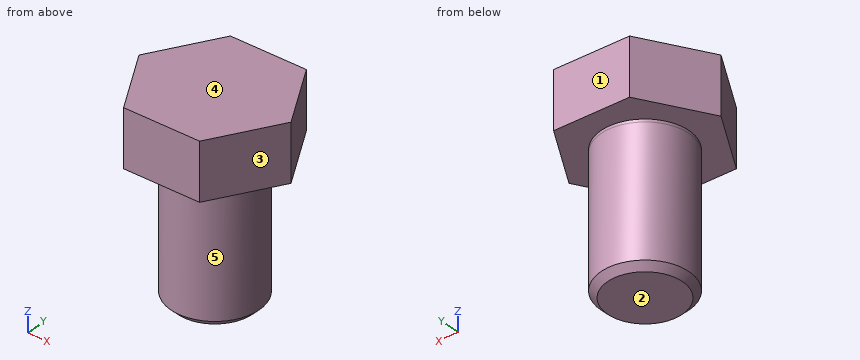
Solid Edge part; units mm, degrees
sketch "Sketch1" plane through (0, 0, 0) normal (0, 0, 1) x (1, 0, 0)
  circle A0 centre (0, 0) radius 13.92
extrude "Protrusion1" add sketch "Sketch1" along normal blind 10.32
sketch "Sketch2" plane through (0, 0, 0) normal (0, 0, -1) x (1, 0, 0)
  circle A0 centre (0, 0) radius 8
extrude "Protrusion2" add sketch "Sketch2" along normal blind 25
sketch "Sketch3" plane through (0, 0, -25) normal (0, 0, -1) x (1, 0, 0)
  circle A0 centre (0, 0) radius 7.9997
extrude "Cutout1" cut sketch "Sketch3" against normal blind 24.5 flip side to cut
chamfer "Chamfer_1" distance 1.2 angle 45 1 edges at (-7.9997, 0, -25)
sketch "Sketch4" plane through (0, 0, 10.32) normal (0, 0, 1) x (1, 0, 0)
  line L0 (-7.0545, 12) -> (7.0545, 12)
extrude "Cutout2" cut sketch "Sketch4" against normal up to next material side at (0, 12.05, 10.32)
pattern_circular "Pattern1" count 6 over 360 about axis through (0, 0, 10.32) along (0, 0, 1) of "Cutout2"
properties part number "118416" material "Stainless Steel, 304"
Input: part model. Units: mm. Frame: model coordinates. Face numbers are marked on the shaded views. A direction names the side the tool comes from. Coordinates: 2 decimals unless noted, no trailing zeros. Loops run counter-clockwise (first coordinate to the right, second up) from the corner with the lowest first, then second, coordinate; pieces in that order, holes last. Notation, with made-up numbers: (-28, 62.25) - (-3, 62.25) arc R14 cw to (-3, 84.25) - close; hole circle Ø4 at (31, 13). An arc over 180 degrees is marked (long way). Answer in a Markdown table with one row per item.
(1) Cut plane C-C on y = -9. Output: boundary loops of the cut face in (x, z), plus the area to 3 significant figures.
Model answer:
| item | result |
|---|---|
| outline | (-8.66, 0) - (8.66, 0) - (8.66, 10.32) - (-8.66, 10.32) - close |
| area | 179 mm² |
(2) Set-up query: the marked faces 4 and 5. Return all of +Z, -Z, +X, -X, +Y, -Y with unobstructed straight access to the full face (end or side cutting, diameter ignored); none if empty.
Model answer:
| item | result |
|---|---|
| face 4 | +Z, +X, -X, +Y, -Y |
| face 5 | -Z |
(3) Cut plane D-D on z = -4. Output: boundary loops of the cut face in (x, y), plus the area to 3 significant figures.
Model answer:
| item | result |
|---|---|
| outline | circle Ø16 at (0, 0) |
| area | 201 mm² |
(4) Pin query (flat end, axial travel): P1, Ø3, axis at y = -5, z = 2.5, coming from the +X side; P2, Ø12, axis at y = -2, z = -9.5, coming from the -X side; P3, Ø10, axis at x = -10.5, z = -15.5, coming from the +Y side. Return the tip coordinate at first contact, or that it passes through.
Model answer:
| item | result |
|---|---|
| P1 | stops at x = 11.84 |
| P2 | stops at x = -8 |
| P3 | stops at y = 5.81 |
(5) Mould query, pull axis Y, two halves, no side actions, for the marked faces 1, 2 and 3. Classes: pulls with the +Y half, pulls with the -Y half, needs draft (parallel to the pull), parting line crosses it, or undercut.
Model answer:
| item | result |
|---|---|
| face 1 | pulls with the +Y half |
| face 2 | needs draft |
| face 3 | pulls with the -Y half |
(6) Cut plane B-B on z = 2. Output: boundary loops of the cut face in (x, y), plus the area to 3 significant figures.
Model answer:
| item | result |
|---|---|
| outline | (-13.86, 0) - (-6.93, -12) - (6.93, -12) - (13.86, 0) - (6.93, 12) - (-6.93, 12) - close |
| area | 499 mm² |
(7) Material intervals for L1, parallel to Z at x = 9.25, y = 2.25; L2, parallel to X at y = 0.25, z = -1.5; L3, parallel to X at y = -5.25, z = -2, sorted ascending. Write a range as from..to.
Model answer:
| item | result |
|---|---|
| L1 | z = 0..10.32 |
| L2 | x = -8..8 |
| L3 | x = -6.04..6.04 |
